Geometry check sheet. Reference: drawing and pictorial views, mm from the part's lowest x, y, z. A direction names the side the tool comes from. Round coordinates to 2 decimals unless told otherwise and drop trailing zeros. Order: outer loops, then holes, each group sorted by start corner. A loop starts at its lowest first (then second) coordinate and runs counter-clockwise, first axis right, second up.
Q1. Depth check by flat-ended pin: P1, Ø1, axis at y = 22, z = 2.5, coming from the -X side. Enter the tip coordinate at first touch or a pass-through.
Q2. Cross-section at C-C on x = 0.8. Record the cut outline in (y, z) (1 decimal).
Q3. Set-up check for the marked faces 1 and 2: record each of +Z, -Z, +X, -X, +Y, -Y from which the full face is reachable in a straight line by a thin tool's end or side.
Q4. Cross-section at B-B on z = 5.75. Record the cut outline in (x, y).
Q5. Scan lines: probe 1 along X at (y, z) = (47, 3); probe 2 along Y at (x, z) = (4.5, 4.25); probe 3 along Z at (x, y) = (2.9, 21.5). Record each from-to range of solid material in increasing order.
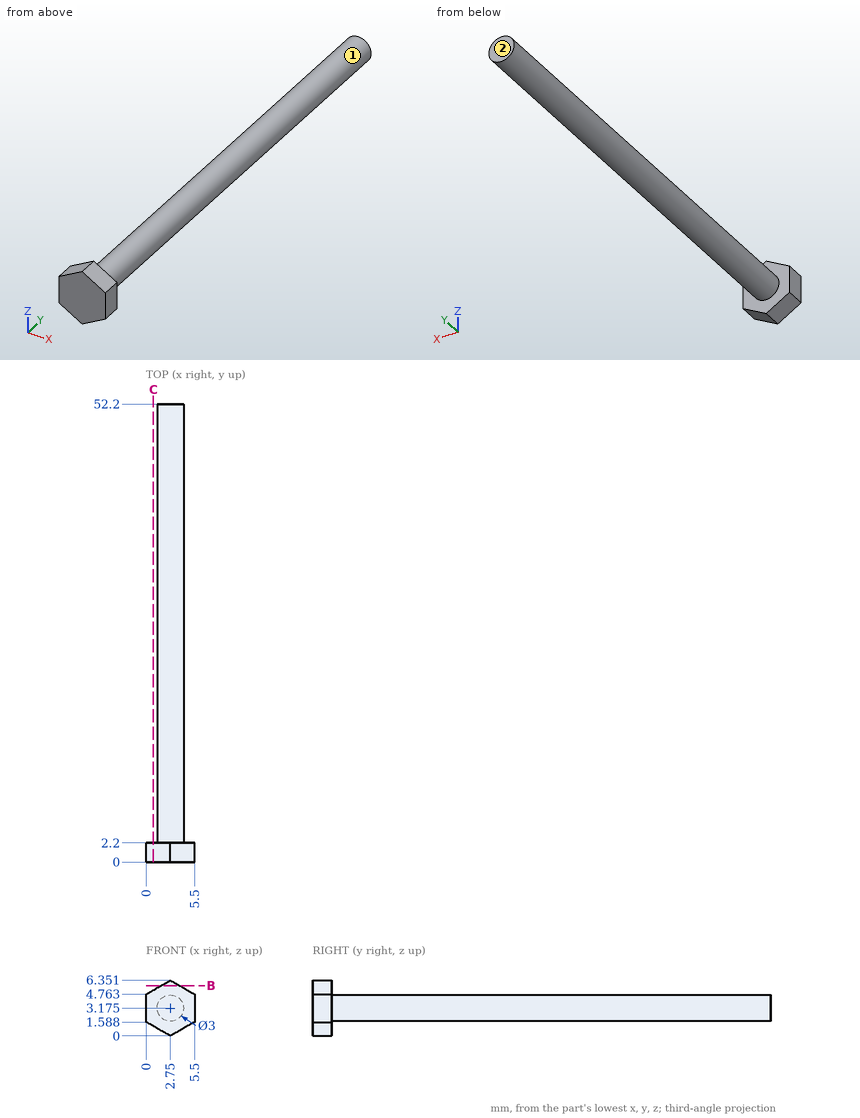
Results found:
1. P1: stops at x = 1.26
2. outline: (0, 1.1) - (2.2, 1.1) - (2.2, 5.2) - (0, 5.2) - close
3. face 1: +Y
3. face 2: +Z, -Z, +X, -X, +Y
4. outline: (1.71, 0) - (3.79, 0) - (3.79, 2.2) - (1.71, 2.2) - close
5. probe 1: x = 1.26 to 4.24
5. probe 2: y = 0 to 2.2
5. probe 3: z = 1.68 to 4.67
